Source: CAD feature listing. Evaluate the final solid. Frame: model axes, mm. Face numbers are marked on the shaded views. A direction names the side the tool comes from. Round coordinates to 2 decimals unless told otherwise and drop trailing zeros. Order: outer loops, then holes, each group sorted by start corner. A loop starts at its lowest first (then second) coordinate and runs counter-clockwise, first axis right, second up. Notation, with made-up numbers: (64.25, 24.5) -> (97.25, 24.5) arc R20 cw to (97.25, 34.5) -> close; hole circle Ø4 at (-2.5, 20.5). An arc over 180 degrees is marked (long way). Write item = value, one per line. Start each with the question number.
(1) Cut plane A-A on y = -22.5. Return the cut outline in (x, z).
(2) Reachability of the marked faces 1, 2 and 3 from +Z, -Z, +X, -X, +Y, -Y: full face, straight path, thin tool, end or side. Return the list, or none.
(3) Ray query, line 1 (Y direction, x = 18, z = 13.25); line 2 (Z direction, x = 15, y = -27) (3 decimals); line 3 (Z direction, x = -11, y = -22). Return the intervals inside material, ascending.
(4) Draft query along Y for the marked faces 4, 5, 6 and 7. Return one class per face: released by +Y, released by -Y, zero draft, split by the parting line, or undercut.
(5) Cut plane C-C on x = -18.6. Return the cut outline in (y, z), then the cut area to 3 significant figures.
(6) Contact query for flat-ended pins moving along their axis: pin 1 Ø3.5 at (x, z) = (15, 7.5) entering from +Y; pin 2 Ø10 at (x, y) = (11, 14) entering from +Z; pin 3 Ø6 at (x, y) = (-12.5, 0) entering from +Z; pin 4 Ø3.5 at (x, z) = (7, 27.5) entering from -Y. Output: stop coordinate, or through.
(7) Cut plane D-D on y = 20. Return the cut outline in (x, z).
(8) Cut plane B-B on x = -7.5. Return the cut outline in (y, z).
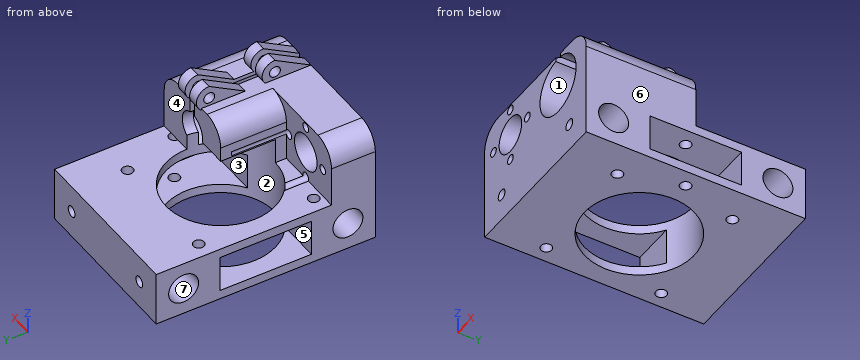
from build123d import *

# Parameters (mm, degrees)
SKETCH1_W           = 45
SKETCH1_H           = 60
BOSS_EXTRUDE1_DEPTH = 15
SKETCH2_R           = 4.1
SKETCH2_W           = 10
SKETCH2_H           = 25
CUT_EXTRUDE1_DEPTH  = 46
SKETCH3_W           = 17
SKETCH3_H           = 12
BOSS_EXTRUDE2_DEPTH = 45
SKETCH4_W           = 25
SKETCH4_H           = 17
BOSS_EXTRUDE3_DEPTH = 18
SKETCH5_W           = 2
SKETCH5_H           = 30
CUT_EXTRUDE2_DEPTH  = 5
SKETCH6_R           = 4.5
CUT_EXTRUDE3_DEPTH  = 61
SKETCH7_R           = 8
SKETCH7_R_2         = 5
SKETCH7_R_3         = 1.25
CUT_EXTRUDE4_DEPTH  = 27
SKETCH8_R           = 15
SKETCH8_R_2         = 1.5
CUT_EXTRUDE5_DEPTH  = 22
FILLET1_R           = 6
SKETCH9_R           = 1.5
CUT_EXTRUDE6_DEPTH  = 15
SKETCH10_R          = 1.5
CUT_EXTRUDE7_DEPTH  = 5
CUT_EXTRUDE8_START  = -60
SKETCH10_2_R        = 1.5
CUT_EXTRUDE8_DEPTH  = 5
SKETCH12_R          = 1.5
BOSS_EXTRUDE4_DEPTH = 3
BOSS_EXTRUDE5_START = 2
SKETCH12_3_R        = 1.5
BOSS_EXTRUDE5_DEPTH = 3


with BuildPart() as part:
    # Sketch1 → Boss-Extrude1 (new body)
    with BuildSketch(Plane.XY):
        Rectangle(SKETCH1_W, SKETCH1_H)
    extrude(amount=BOSS_EXTRUDE1_DEPTH)

    # Sketch2 → Cut-Extrude1 (cut, through all)
    with BuildSketch(Plane(origin=(22.5, 0, 0), x_dir=(0, 0, -1), z_dir=(1, 0, 0))):
        with Locations((-7.5, 22.5)):
            Circle(SKETCH2_R)
        with Locations((-7.5, -22.5)):
            Circle(SKETCH2_R)
        with Locations((-7.5, 0)):
            Rectangle(SKETCH2_W, SKETCH2_H)
    extrude(amount=-CUT_EXTRUDE1_DEPTH, mode=Mode.SUBTRACT)

    # Sketch3 → Boss-Extrude2 (add)
    with BuildSketch(Plane.ZY.offset(22.5)):
        with Locations((23.5, -24)):
            Rectangle(SKETCH3_W, SKETCH3_H)
    extrude(amount=-BOSS_EXTRUDE2_DEPTH)

    # Sketch4 → Boss-Extrude3 (add)
    with BuildSketch(Plane(origin=(0, -18, 0), x_dir=(1, 0, 0), z_dir=(0, 1, 0))):
        with Locations((10, -23.5)):
            Rectangle(SKETCH4_W, SKETCH4_H)
    extrude(amount=BOSS_EXTRUDE3_DEPTH)

    # Sketch5 → Cut-Extrude2 (cut)
    with BuildSketch(Plane.XY.offset(32)):
        with Locations((10, -15)):
            Rectangle(SKETCH5_W, SKETCH5_H)
    extrude(amount=-CUT_EXTRUDE2_DEPTH, mode=Mode.SUBTRACT)

    # Sketch6 → Cut-Extrude3 (cut, through all)
    with BuildSketch(Plane.XZ.offset(30)):
        with Locations((10, 23)):
            Circle(SKETCH6_R)
    extrude(amount=-CUT_EXTRUDE3_DEPTH, mode=Mode.SUBTRACT)

    # Sketch7 → Cut-Extrude4 (cut)
    with BuildSketch(Plane.XZ.offset(30)):
        with Locations((10, 23)):
            Circle(SKETCH7_R)
        with Locations((-11.1, 23)):
            Circle(SKETCH7_R_2)
        with Locations((-3.6, 23)):
            Circle(SKETCH7_R_3)
        with Locations((-11.1, 30.5)):
            Circle(SKETCH7_R_3)
        with Locations((-11.1, 15.5)):
            Circle(SKETCH7_R_3)
        with Locations((-18.6, 23)):
            Circle(SKETCH7_R_3)
    extrude(amount=-CUT_EXTRUDE4_DEPTH, mode=Mode.SUBTRACT)

    # Sketch8 → Cut-Extrude5 (cut)
    with BuildSketch(Plane(origin=(0, 0, 0), x_dir=(-1, 0, 0), z_dir=(0, 0, -1))):
        with Locations((2.5, 0)):
            Circle(SKETCH8_R)
        with Locations((18.25, 15.75)):
            Circle(SKETCH8_R_2)
        with Locations((-13.25, 15.75)):
            Circle(SKETCH8_R_2)
        with Locations((-13.25, -15.75)):
            Circle(SKETCH8_R_2)
        with Locations((18.25, -15.75)):
            Circle(SKETCH8_R_2)
    extrude(amount=-CUT_EXTRUDE5_DEPTH, mode=Mode.SUBTRACT)

    # Fillet1
    fillet1_edges = [part.edges().sort_by_distance(p)[0] for p in [
        (-22.5, -24, 32),
        (-2.5, -9, 32),
        (22.5, -15, 32),
    ]]
    fillet(fillet1_edges, radius=FILLET1_R)

    # Sketch9 → Cut-Extrude6 (cut)
    with BuildSketch(Plane(origin=(0, 0, 0), x_dir=(-1, 0, 0), z_dir=(0, 0, -1))):
        with Locations((-18, 0)):
            Circle(SKETCH9_R)
    extrude(amount=-CUT_EXTRUDE6_DEPTH, mode=Mode.SUBTRACT)

    # Sketch10 → Cut-Extrude7 (cut)
    with BuildSketch(Plane(origin=(0, 30, 0), x_dir=(1, 0, 0), z_dir=(0, 1, 0))):
        with Locations((-15, -7.5)):
            Circle(SKETCH10_R)
        with Locations((15, -7.5)):
            Circle(SKETCH10_R)
    extrude(amount=-CUT_EXTRUDE7_DEPTH, mode=Mode.SUBTRACT)

    # Sketch10<2> → Cut-Extrude8 (cut)
    with BuildSketch(Plane(origin=(0, 30, 0), x_dir=(1, 0, 0), z_dir=(0, 1, 0)).offset(CUT_EXTRUDE8_START)):
        with Locations((-15, -7.5)):
            Circle(SKETCH10_2_R)
        with Locations((15, -7.5)):
            Circle(SKETCH10_2_R)
    extrude(amount=CUT_EXTRUDE8_DEPTH, mode=Mode.SUBTRACT)

    # Sketch12 → Boss-Extrude4 (add)
    with BuildSketch(Plane(origin=(9, 0, 0), x_dir=(0, 0, -1), z_dir=(1, 0, 0))):
        with BuildLine():
            Line((-32, -30), (-37.75, -20.113140033))
            ThreePointArc((-37.75, -20.113140033), (-34.822445965, -16.660270847), (-30.937253933, -18.983665157))
            Line((-30.937253933, -18.983665157), (-30.937253933, -30))
            Line((-30.937253933, -30), (-32, -30))
        make_face()
        with Locations((-34.25, -20.113140033)):
            Circle(SKETCH12_R, mode=Mode.SUBTRACT)
        with BuildLine():
            Line((-32, -12), (-37.75, -2.113140033))
            ThreePointArc((-37.75, -2.113140033), (-34.822445965, 1.339729153), (-30.937253933, -0.983665157))
            Line((-30.937253933, -0.983665157), (-30.937253933, -12))
            Line((-30.937253933, -12), (-32, -12))
        make_face()
        with Locations((-34.25, -2.113140033)):
            Circle(SKETCH12_R, mode=Mode.SUBTRACT)
    extrude(amount=-BOSS_EXTRUDE4_DEPTH)

    # Sketch12<3> → Boss-Extrude5 (add)
    with BuildSketch(Plane(origin=(9, 0, 0), x_dir=(0, 0, -1), z_dir=(1, 0, 0)).offset(BOSS_EXTRUDE5_START)):
        with BuildLine():
            Line((-32, -30), (-37.75, -20.113140033))
            ThreePointArc((-37.75, -20.113140033), (-34.822445965, -16.660270847), (-30.937253933, -18.983665157))
            Line((-30.937253933, -18.983665157), (-30.937253933, -30))
            Line((-30.937253933, -30), (-32, -30))
        make_face()
        with Locations((-34.25, -20.113140033)):
            Circle(SKETCH12_3_R, mode=Mode.SUBTRACT)
        with BuildLine():
            Line((-32, -12), (-37.75, -2.113140033))
            ThreePointArc((-37.75, -2.113140033), (-34.822445965, 1.339729153), (-30.937253933, -0.983665157))
            Line((-30.937253933, -0.983665157), (-30.937253933, -12))
            Line((-30.937253933, -12), (-32, -12))
        make_face()
        with Locations((-34.25, -2.113140033)):
            Circle(SKETCH12_3_R, mode=Mode.SUBTRACT)
    extrude(amount=BOSS_EXTRUDE5_DEPTH)


solid = part.part
Evaluation:
q1.outline = (-22.5, 0) -> (22.5, 0) -> (22.5, 3.4) -> (-22.5, 3.4) -> close; (-22.5, 11.6) -> (22.5, 11.6) -> (22.5, 26) arc R6 ccw to (16.5, 32) -> (14, 32) -> (14, 36.36) -> (11, 36.36) -> (11, 30.94) arc R8 cw (long way) to (9, 30.94) -> (9, 36.36) -> (6, 36.36) -> (6, 32) -> (-16.5, 32) arc R6 ccw to (-22.5, 26) -> close; hole circle Ø2.5 at (-18.6, 23); hole circle Ø10 at (-11.1, 23); hole circle Ø2.5 at (-11.1, 15.5); hole circle Ø2.5 at (-11.1, 30.5); hole circle Ø2.5 at (-3.6, 23)
q2.face_1 = -Y
q2.face_2 = -Z
q2.face_3 = +X, -X
q3.line_1 = -30 to -1.5, 1.5 to 30
q3.line_2 = 0 to 6, 9 to 16.755, 29.245 to 32
q3.line_3 = 0 to 3.43, 11.57 to 14.25, 16.75 to 18, 28 to 29.25, 31.75 to 32
q4.face_4 = released by +Y
q4.face_5 = undercut
q4.face_6 = zero draft
q4.face_7 = undercut
q5.outline = (-30, 0) -> (-17.21, 0) -> (-17.21, 15) -> (-18, 15) -> (-18, 21.75) -> (-30, 21.75) -> close; (-30, 24.25) -> (-18, 24.25) -> (-18, 31.62) -> (-30, 31.62) -> close; (-14.29, 0) -> (14.29, 0) -> (14.29, 15) -> (-14.29, 15) -> close; (17.21, 0) -> (30, 0) -> (30, 15) -> (17.21, 15) -> close; hole circle Ø8.2 at (-22.5, 7.5); hole (-12.5, 2.5) -> (12.5, 2.5) -> (12.5, 12.5) -> (-12.5, 12.5) -> close; hole circle Ø8.2 at (22.5, 7.5)
q5.area = 626 mm^2
q6.pin_1 = 30
q6.pin_2 = 15
q6.pin_3 = through
q6.pin_4 = -3
q7.outline = (-22.5, 0) -> (22.5, 0) -> (22.5, 4.25) -> (-22.5, 4.25) -> close; (-22.5, 10.75) -> (22.5, 10.75) -> (22.5, 15) -> (-22.5, 15) -> close
q8.outline = (-30, 0) -> (-14.14, 0) -> (-14.14, 15) -> (-18, 15) -> (-18, 19.53) -> (-30, 19.53) -> close; (-30, 26.47) -> (-18, 26.47) -> (-18, 32) -> (-30, 32) -> close; (14.14, 0) -> (30, 0) -> (30, 15) -> (14.14, 15) -> close; hole circle Ø8.2 at (-22.5, 7.5); hole circle Ø8.2 at (22.5, 7.5)
